```python
from build123d import *

# Parameters (mm, degrees)
SKETCH_1_R      = 2
SKETCH_1_R_2    = 41
SKETCH_1_R_3    = 1.45
EXTRUDE_1_DEPTH = 6


with BuildPart() as part:
    # 草图1 → 凸台-拉伸1 (new body)
    with BuildSketch(Plane(origin=(0, 0, 0), x_dir=(1, 0, 0), z_dir=(0, 1, 0))):
        with BuildLine():
            Line((-77.023496261, 50), (77.023496261, 50))
            ThreePointArc((77.023496261, 50), (78.005849606, 49.902548511), (78.949910233, 49.613992762))
            ThreePointArc((78.949910233, 49.613992762), (112, 0), (78.949910233, -49.613992762))
            ThreePointArc((78.949910233, -49.613992762), (78.005849606, -49.902548511), (77.023496261, -50))
            Line((77.023496261, -50), (-77.023496261, -50))
            ThreePointArc((-77.023496261, -50), (-78.005849606, -49.902548511), (-78.949910233, -49.613992762))
            ThreePointArc((-78.949910233, -49.613992762), (-112, 0), (-78.949910233, 49.613992762))
            ThreePointArc((-78.949910233, 49.613992762), (-78.005849606, 49.902548511), (-77.023496261, 50))
        make_face()
        with Locations(Location((60, 45, 0), (0, 0, 270))):
            Circle(SKETCH_1_R, mode=Mode.SUBTRACT)
        with Locations(Location((21.02885683, 22.5, 0), (0, 0, 270))):
            Circle(SKETCH_1_R, mode=Mode.SUBTRACT)
        with Locations(Location((21.02885683, -22.5, 0), (0, 0, 270))):
            Circle(SKETCH_1_R, mode=Mode.SUBTRACT)
        with Locations(Location((60, -45, 0), (0, 0, 270))):
            Circle(SKETCH_1_R, mode=Mode.SUBTRACT)
        with Locations(Location((98.97114317, -22.5, 0), (0, 0, 270))):
            Circle(SKETCH_1_R, mode=Mode.SUBTRACT)
        with Locations(Location((98.97114317, 22.5, 0), (0, 0, 270))):
            Circle(SKETCH_1_R, mode=Mode.SUBTRACT)
        with Locations(Location((60, 0, 0), (0, 0, 270))):
            Circle(SKETCH_1_R_2, mode=Mode.SUBTRACT)
        with Locations(Location((-60, 0, 0), (0, 0, 90))):
            Circle(SKETCH_1_R_2, mode=Mode.SUBTRACT)
        with Locations(Location((-21.02885683, -22.5, 0), (0, 0, 90))):
            Circle(SKETCH_1_R, mode=Mode.SUBTRACT)
        with Locations(Location((-21.02885683, 22.5, 0), (0, 0, 90))):
            Circle(SKETCH_1_R, mode=Mode.SUBTRACT)
        with Locations(Location((-60, 45, 0), (0, 0, 90))):
            Circle(SKETCH_1_R, mode=Mode.SUBTRACT)
        with Locations(Location((-98.97114317, 22.5, 0), (0, 0, 90))):
            Circle(SKETCH_1_R, mode=Mode.SUBTRACT)
        with Locations(Location((-98.97114317, -22.5, 0), (0, 0, 90))):
            Circle(SKETCH_1_R, mode=Mode.SUBTRACT)
        with Locations(Location((-60, -45, 0), (0, 0, 90))):
            Circle(SKETCH_1_R, mode=Mode.SUBTRACT)
        with Locations(Location((-5, 45, 0), (0, 0, 270))):
            Circle(SKETCH_1_R_3, mode=Mode.SUBTRACT)
        with Locations(Location((5, 45, 0), (0, 0, 270))):
            Circle(SKETCH_1_R_3, mode=Mode.SUBTRACT)
        with Locations(Location((-5, 0, 0), (0, 0, 270))):
            Circle(SKETCH_1_R_3, mode=Mode.SUBTRACT)
        with Locations(Location((5, 0, 0), (0, 0, 270))):
            Circle(SKETCH_1_R_3, mode=Mode.SUBTRACT)
        with Locations(Location((-5, -45, 0), (0, 0, 270))):
            Circle(SKETCH_1_R_3, mode=Mode.SUBTRACT)
        with Locations(Location((5, -45, 0), (0, 0, 270))):
            Circle(SKETCH_1_R_3, mode=Mode.SUBTRACT)
        with Locations(Location((-15, 35, 0), (0, 0, 270))):
            Circle(SKETCH_1_R_3, mode=Mode.SUBTRACT)
        with Locations(Location((15, 35, 0), (0, 0, 90))):
            Circle(SKETCH_1_R_3, mode=Mode.SUBTRACT)
        with Locations(Location((-15, -45, 0), (0, 0, 270))):
            Circle(SKETCH_1_R_3, mode=Mode.SUBTRACT)
        with Locations(Location((-25, -45, 0), (0, 0, 270))):
            Circle(SKETCH_1_R_3, mode=Mode.SUBTRACT)
        with Locations(Location((25, -45, 0), (0, 0, 90))):
            Circle(SKETCH_1_R_3, mode=Mode.SUBTRACT)
        with Locations(Location((15, -45, 0), (0, 0, 90))):
            Circle(SKETCH_1_R_3, mode=Mode.SUBTRACT)
        with BuildLine():
            Line((-3.5, -7.5), (-3.5, -37))
            ThreePointArc((-3.5, -37), (-3.939339828, -38.060660172), (-5, -38.5))
            Line((-5, -38.5), (-23.60480801, -38.5))
            ThreePointArc((-23.60480801, -38.5), (-24.992980593, -37.568310548), (-24.656692171, -35.930635838))
            ThreePointArc((-24.656692171, -35.930635838), (-15.049616268, -22.795240783), (-10.129021878, -7.283236994))
            ThreePointArc((-10.129021878, -7.283236994), (-9.625800595, -6.36528759), (-8.644766576, -6))
            Line((-8.644766576, -6), (-5, -6))
            ThreePointArc((-5, -6), (-3.939339828, -6.439339828), (-3.5, -7.5))
        make_face(mode=Mode.SUBTRACT)
        with BuildLine():
            Line((5, -6), (8.644766576, -6))
            ThreePointArc((8.644766576, -6), (9.625800595, -6.36528759), (10.129021878, -7.283236994))
            ThreePointArc((10.129021878, -7.283236994), (15.049616268, -22.795240783), (24.656692171, -35.930635838))
            ThreePointArc((24.656692171, -35.930635838), (24.992980593, -37.568310548), (23.60480801, -38.5))
            Line((23.60480801, -38.5), (5, -38.5))
            ThreePointArc((5, -38.5), (3.939339828, -38.060660172), (3.5, -37))
            Line((3.5, -37), (3.5, -7.5))
            ThreePointArc((3.5, -7.5), (3.939339828, -6.439339828), (5, -6))
        make_face(mode=Mode.SUBTRACT)
        with BuildLine():
            Line((-15.984548168, 29), (-4.5, 29))
            ThreePointArc((-4.5, 29), (-3.439339828, 28.560660172), (-3, 27.5))
            Line((-3, 27.5), (-3, 6.5))
            ThreePointArc((-3, 6.5), (-3.439339828, 5.439339828), (-4.5, 5))
            Line((-4.5, 5), (-8.508641502, 5))
            ThreePointArc((-8.508641502, 5), (-9.500661686, 5.374879583), (-9.996831054, 6.312138728))
            ThreePointArc((-9.996831054, 6.312138728), (-12.518977702, 16.90303291), (-17.256671053, 26.705202312))
            ThreePointArc((-17.256671053, 26.705202312), (-17.296454516, 28.227256306), (-15.984548168, 29))
        make_face(mode=Mode.SUBTRACT)
        with BuildLine():
            Line((15.984548168, 29), (4.5, 29))
            ThreePointArc((4.5, 29), (3.439339828, 28.560660172), (3, 27.5))
            Line((3, 27.5), (3, 6.5))
            ThreePointArc((3, 6.5), (3.439339828, 5.439339828), (4.5, 5))
            Line((4.5, 5), (8.508641502, 5))
            ThreePointArc((8.508641502, 5), (9.500661686, 5.374879583), (9.996831054, 6.312138728))
            ThreePointArc((9.996831054, 6.312138728), (12.518977702, 16.90303291), (17.256671053, 26.705202312))
            ThreePointArc((17.256671053, 26.705202312), (17.296454516, 28.227256306), (15.984548168, 29))
        make_face(mode=Mode.SUBTRACT)
    extrude(amount=EXTRUDE_1_DEPTH)


solid = part.part
```
Design review of the part built by this model. Coordinates are the model's own, in mm. A direction names the side the tool comes from. Give positions to 0.01 mm unless a question says otherwise; leave off trailing zeros. Loops run counter-clockwise (first coordinate to the right, second up) from the corner with the lowest first, then second, coordinate; pieces in that order, holes last. Notation, with made-up numbers: M 71.5,-9 L 122.5,-9 A6 cw 122.5,2 Z; hole C -31.75,53.25 d9. An arc over 180 degrees is marked long. Return JSON: item names as keys, results as strings. Group by question number.
Item 1: Mouldability with a two-part tool opening along Z and no side actions: class faces 3 (the flat face through (-1, 3, -50)), 4 (the flat face through (3, 3, -17)), 5 (the cylindrical face through (-111.993, 2.958, 0.885)) as released by +Z, released by -Z, zero draft, split by the parting line, or undercut.
Item 2: For probe 1 along X at (y, z) = (0.4, -2); probe 2 along Z at (x, y) = (7.5, 4.45); probe 3 along X at (y, z) = (1.8, 0), list the stretches that pass through material, from the lowest coordinate up.
Item 3: Tool access review of faces 1 (the flat face through (2, 0, -1)), 2 (the flat face through (-14, 3, 38.5)): name each direction out of +Z, -Z, +X, -X, +Y, -Y from which nothing blocks a thin tool from reaching the whole face with its end or side.
Item 4: We need section B-B (z = 12.5). Give the boundary of the cut face in (x, y).
Item 5: Insertion check: pin 1 Ø2.5 at (x, z) = (-5, 0) entering from -Y; pin 2 Ø1.8 at (y, z) = (2, 23) entering from +X; pin 3 Ø3 at (y, z) = (4, 32) entering from +X. Each pin has a flat end and moves straight along its axis. Give the tip position at first contact, or say it passes through.
Item 6: We need section C-C (y = 3.2). Give the number of separate pieces and of enclosed holes in the cut face, and give its area (3 significant figures).
Item 7: We need section A-A (x = -60). Give the boundary of the cut face in (y, z).
Output:
{
 "1": {"face 3": "released by -Z", "face 4": "undercut", "face 5": "split by the parting line"},
 "2": {"probe 1": "x = -111.96 to -100.95, -19.05 to 19.05, 100.95 to 111.96", "probe 2": "z = -50 to -29, -5 to 6, 38.5 to 50", "probe 3": "x = -112 to -101, -19 to -6.45, -3.55 to 3.55, 6.45 to 19, 101 to 112"},
 "3": {"face 1": "+Z, -Z, +X, -X, -Y", "face 2": "+Y, -Y"},
 "4": {"outline": "M -110.53,0 L -99.05,0 L -99.05,6 L -110.53,6 Z; M -20.95,0 L -11.17,0 L -11.17,6 L -20.95,6 Z; M -3.5,0 L 3.5,0 L 3.5,6 L -3.5,6 Z; M 11.17,0 L 20.95,0 L 20.95,6 L 11.17,6 Z; M 99.05,0 L 110.53,0 L 110.53,6 L 99.05,6 Z"},
 "5": {"pin 1": "passes through", "pin 2": "stops at x = 107.25", "pin 3": "stops at x = 102.51"},
 "6": {"separate pieces": "1", "enclosed holes": "30", "area": "8,450 mm^2"},
 "7": {"outline": "M 0,-50 L 6,-50 L 6,-47 L 0,-47 Z; M 0,-43 L 6,-43 L 6,-41 L 0,-41 Z; M 0,41 L 6,41 L 6,43 L 0,43 Z; M 0,47 L 6,47 L 6,50 L 0,50 Z"}
}
